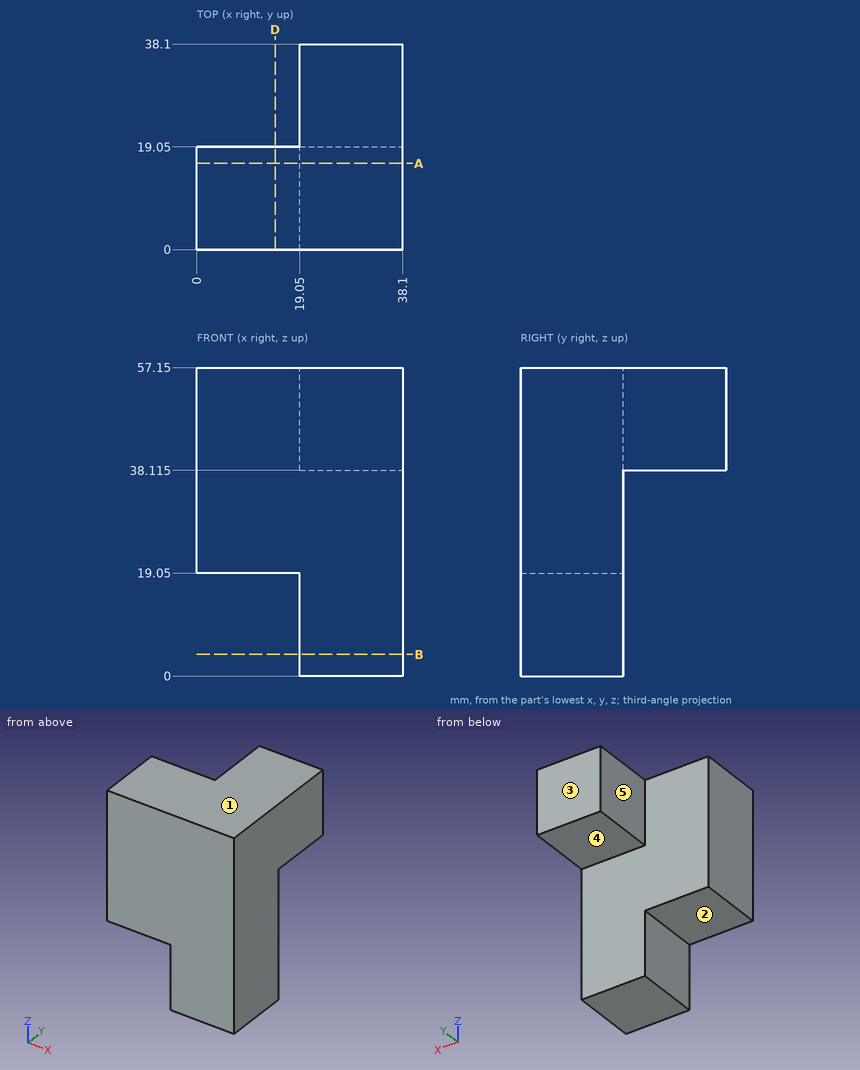
For this review, use the dimensioned drawing (mm, ordinates from the lowest corner) and the shaded views. A direction names the side the tool comes from. Give positions to 0.01 mm unless a question says otherwise; leave off trailing zeros. Write each loop counter-clockwise with the first axis right and the second up, starting at its lowest first coordinate (ties: lowest second). Pieces come first, ordered by that corner, then holes. Notation, with made-up numbers: M 37,11.25 L 94,11.25 A30 ccw 94,33.25 Z; hole C 57,-30.5 d7. An arc over 180 degrees is marked long. Write item = value, one per line. Start each with the question number.
Q1. For line 1 (Y direction, x = 15, z = 33); line 2 (Z direction, x = 14.5, y = 13); line 3 (X direction, y = 29.5, z = 41.5), list the stretches that pass through material, from the lowest coordinate up.
Q2. We need section B-B (z = 4). State the section outline as (x, y) points, plus the area to 3 significant figures.
Q3. We need section A-A (y = 16). State the section outline as (x, z) points, plus the area to 3 significant figures.
Q4. Machinability: for the marked faces 1, 2, 3, 4 and 5, which of the approach directions +Z, -Z, +X, -X, +Y, -Y give a long, thin tool a straight path to every point of the face, cutting with its end or side? Answer none if there is none.
Q5. Clearance check with flat-ended pins moving along their axes: pin 1 (2 mm diameter, centred on x = 27.5, z = 32.5, fed in from +Y); pin 2 (5.5 mm diameter, centred on x = 11.5, y = 9, fed in from -Z); pin 3 (21 mm diameter, centred on y = 30.5, z = 48.5, fed in from -X); pin 4 (12 mm diameter, centred on y = 30, z = 19, fed in from -X). State where each tip first meets the part, or that it passes through.
Q6. We need section D-D (x = 14.5). State the section outline as (y, z) points.
Result set:
q1.line_1 = 0 to 19.05
q1.line_2 = 19.05 to 57.15
q1.line_3 = 19.05 to 38.1
q2.outline = M 19.05,0 L 38.1,0 L 38.1,19.05 L 19.05,19.05 Z
q2.area = 363 mm2
q3.outline = M 0,19.05 L 19.05,19.05 L 19.05,0 L 38.1,0 L 38.1,57.15 L 0,57.15 Z
q3.area = 1,810 mm2
q4.face_1 = +Z, +X, -X, +Y, -Y
q4.face_2 = -Z, -X, +Y, -Y
q4.face_3 = +Z, -Z, +X, -X, +Y
q4.face_4 = -Z, +X, -X, +Y
q4.face_5 = +Z, -Z, -X, +Y
q5.pin_1 = 19.05
q5.pin_2 = 19.05
q5.pin_3 = 19.05
q5.pin_4 = through
q6.outline = M 0,19.05 L 19.05,19.05 L 19.05,57.15 L 0,57.15 Z
